Can you work these out from the model? Positions are in its coordinate system, mm. A direction names the side the tool comes from. Give positions to 0.01 mm unless a question says otherwise; leave off trailing zeros. Loops run counter-clockwise (first coordinate to the right, second up) from the corner with the lowest first, then second, coordinate; pieces in that order, holes last. Notation, with made-up numbers: (-23.5, 76) - (-0.5, 76) arc R37 cw to (-0.5, 112) - close; hole circle Ø3 at (-34.5, 4.25). An arc over 180 degrees is marked (long way). Answer as a JSON object with one key per item and string values.
```python
from build123d import *

# Parameters (mm, degrees)
SKETCH1_R           = 8.5
BOSS_EXTRUDE1_DEPTH = 23
SHELL3_T            = -0.3
SKETCH2_R           = 8.2
BOSS_EXTRUDE2_DEPTH = 0.3
SKETCH3_R           = 1.15
BOSS_EXTRUDE3_DEPTH = 1.5
SKETCH4_R           = 2.929639603
SKETCH4_R_2         = 2.629639603
BOSS_EXTRUDE4_DEPTH = 1.5
SKETCH5_R           = 0.75
BOSS_EXTRUDE5_DEPTH = 3.8
CUT_EXTRUDE1_REACH  = 28.842
SKETCH7_R           = 1
SKETCH8_W           = 2.3
SKETCH8_H           = 4
BOSS_EXTRUDE7_DEPTH = 2.85


with BuildPart() as part:
    # Sketch1 → Boss-Extrude1 (new body)
    with BuildSketch(Plane(origin=(0, 0, 0), x_dir=(1, 0, 0), z_dir=(0, 1, 0))):
        with Locations(Location((0, 0, 0), (0, 0, 270))):
            Circle(SKETCH1_R)
    extrude(amount=BOSS_EXTRUDE1_DEPTH)

    # Shell3
    shell3_openings = [part.faces().sort_by_distance(p)[0] for p in [
        (0, 0, 0),
    ]]
    offset(amount=SHELL3_T, openings=shell3_openings, kind=Kind.INTERSECTION)

    # Sketch2 → Boss-Extrude2 (add)
    with BuildSketch(Plane(origin=(0, 0.5, 0), x_dir=(-1, 0, 0), z_dir=(0, -1, 0))):
        with Locations(Location((0, 0, 0), (0, 0, 90))):
            Circle(SKETCH2_R)
    extrude(amount=-BOSS_EXTRUDE2_DEPTH)

    # Sketch3 → Boss-Extrude3 (add)
    with BuildSketch(Plane.XZ.offset(-0.5)):
        with Locations(Location((0, 0, 0), (0, 0, 270))):
            Circle(SKETCH3_R)
    extrude(amount=BOSS_EXTRUDE3_DEPTH)

    # Sketch4 → Boss-Extrude4 (add)
    with BuildSketch(Plane(origin=(0, 23, 0), x_dir=(1, 0, 0), z_dir=(0, 1, 0))):
        with Locations(Location((0, 0, 0), (0, 0, 270))):
            Circle(SKETCH4_R)
        with Locations(Location((0, 0, 0), (0, 0, 270))):
            Circle(SKETCH4_R_2, mode=Mode.SUBTRACT)
    extrude(amount=BOSS_EXTRUDE4_DEPTH)

    # Sketch5 → Boss-Extrude5 (add)
    with BuildSketch(Plane(origin=(0, 23, 0), x_dir=(1, 0, 0), z_dir=(0, 1, 0))):
        with Locations(Location((0, 0, 0), (0, 0, 90))):
            Circle(SKETCH5_R)
    extrude(amount=BOSS_EXTRUDE5_DEPTH)

    # Sketch7 → Cut-Extrude1 (cut, up to next)
    with BuildSketch(Plane(origin=(0, 23, 0), x_dir=(1, 0, 0), z_dir=(0, 1, 0)), mode=Mode.PRIVATE) as cut_extrude1_sk1:
        with Locations(Location((0, 5, 0), (0, 0, 270))):
            Circle(SKETCH7_R)
    cut_extrude1_tool1 = extrude(cut_extrude1_sk1.sketch, amount=-CUT_EXTRUDE1_REACH, mode=Mode.PRIVATE) & part.part
    # Sketch7 → Cut-Extrude1 (cut, up to next)
    with BuildSketch(Plane(origin=(0, 23, 0), x_dir=(1, 0, 0), z_dir=(0, 1, 0)), mode=Mode.PRIVATE) as cut_extrude1_sk2:
        with Locations(Location((0, -5, 0), (0, 0, 270))):
            Circle(SKETCH7_R)
    cut_extrude1_tool2 = extrude(cut_extrude1_sk2.sketch, amount=-CUT_EXTRUDE1_REACH, mode=Mode.PRIVATE) & part.part
    add(cut_extrude1_tool1.solids().sort_by_distance((0, 23, -5))[0], mode=Mode.SUBTRACT)
    add(cut_extrude1_tool2.solids().sort_by_distance((0, 23, 5))[0], mode=Mode.SUBTRACT)

    # Sketch8 → Boss-Extrude7 (add)
    with BuildSketch(Plane.XZ.offset(-0.5)):
        with Locations((-6, 0)):
            Rectangle(SKETCH8_W, SKETCH8_H)
        with Locations((6, 0)):
            Rectangle(SKETCH8_W, SKETCH8_H)
    extrude(amount=BOSS_EXTRUDE7_DEPTH)


solid = part.part
```
1) Imagine slicing it at B-B on z = -3.25. Write out the boundary of the cut face in (x, y), and give its area (3 significant figures).
Check sheet entries:
{"outline": "(-7.85, 0) - (-7.53, 0) - (-7.53, 0.5) - (7.53, 0.5) - (7.53, 0) - (7.85, 0) - (7.85, 23) - (-7.85, 23) - close; hole (-7.53, 0.8) - (7.53, 0.8) - (7.53, 22.7) - (-7.53, 22.7) - close", "area": "24.0 mm2"}
2) If we mould it in two halves opening along Z, with no side actions, what happens to faces 1 (the cylindrical face through (2.905, 23.74, -0.381)), 2 (the flat face through (0, 22.7, 0)), 3 (the flat face through (6, -2.35, 0))? For each: released by +Z, released by -Z, zero draft, split by the parting line, or undercut.
Check sheet entries:
{"face 1": "split by the parting line", "face 2": "undercut", "face 3": "zero draft"}
3) Which directions (+Z, -Z, +X, -X, +Y, -Y) give clear straight access to the entire face, cutting with the end or side of a thin tool? Please do faces 4 (the flat face through (0, 26.8, 0)), 5 (the flat face through (0.1, 23, 3.7)), 6 (the flat face through (-7.15, -1, 0)), 7 (the flat face through (0, -1, 0)).
Check sheet entries:
{"face 4": "+Z, -Z, +X, -X, +Y", "face 5": "+Y", "face 6": "-Y", "face 7": "+Z, -Z, -Y"}
4) Imagine slicing it at A-A on x = -3.5. Write out the boundary of the cut face in (y, z).
Check sheet entries:
{"outline": "(0, -7.75) - (23, -7.75) - (23, 7.75) - (0, 7.75) - (0, 7.42) - (0.5, 7.42) - (0.5, -7.42) - (0, -7.42) - close; hole (0.8, -7.42) - (22.7, -7.42) - (22.7, 7.42) - (0.8, 7.42) - close"}
5) Imagine slicing it at C-C on y = 17.5. Write out the boundary of the cut face in (x, z).
Check sheet entries:
{"outline": "circle Ø17 at (0, 0); hole circle Ø16.4 at (0, 0)"}
6) Imagine slicing it at D-D on z = -5. Write out the boundary of the cut face in (x, y).
Check sheet entries:
{"outline": "(-6.87, 0) - (-6.5, 0) - (-6.5, 0.5) - (6.5, 0.5) - (6.5, 0) - (6.87, 0) - (6.87, 23) - (1, 23) - (1, 22.7) - (6.5, 22.7) - (6.5, 0.8) - (-6.5, 0.8) - (-6.5, 22.7) - (-1, 22.7) - (-1, 23) - (-6.87, 23) - close"}
7) I need wall thicknesses on L1, parallel to X at y = 23.4, z = 0; L2, parallel to X at y = 0.2, z = 0; L3, parallel to X at y = 12.5, z = 0. Which ranges of each line are inside material? Lowest first, please.
Check sheet entries:
{"L1": "-2.93 to -2.63, -0.75 to 0.75, 2.63 to 2.93", "L2": "-8.5 to -8.2, -7.15 to -4.85, -1.15 to 1.15, 4.85 to 7.15, 8.2 to 8.5", "L3": "-8.5 to -8.2, 8.2 to 8.5"}
8) I'm going to push flat-ended pins straight in: P1, Ø3, axis at x = 6, y = 14.5, coming from the +Z side; P2, Ø4, axis at x = 6.5, y = 19, coming from the -Z side; P3, Ø6, axis at y = 6, z = -5.5, coming from the +X side. Where does each tip first touch, or does it pass through?
Check sheet entries:
{"P1": "z = 7.21", "P2": "z = -7.21", "P3": "x = 8.12"}
